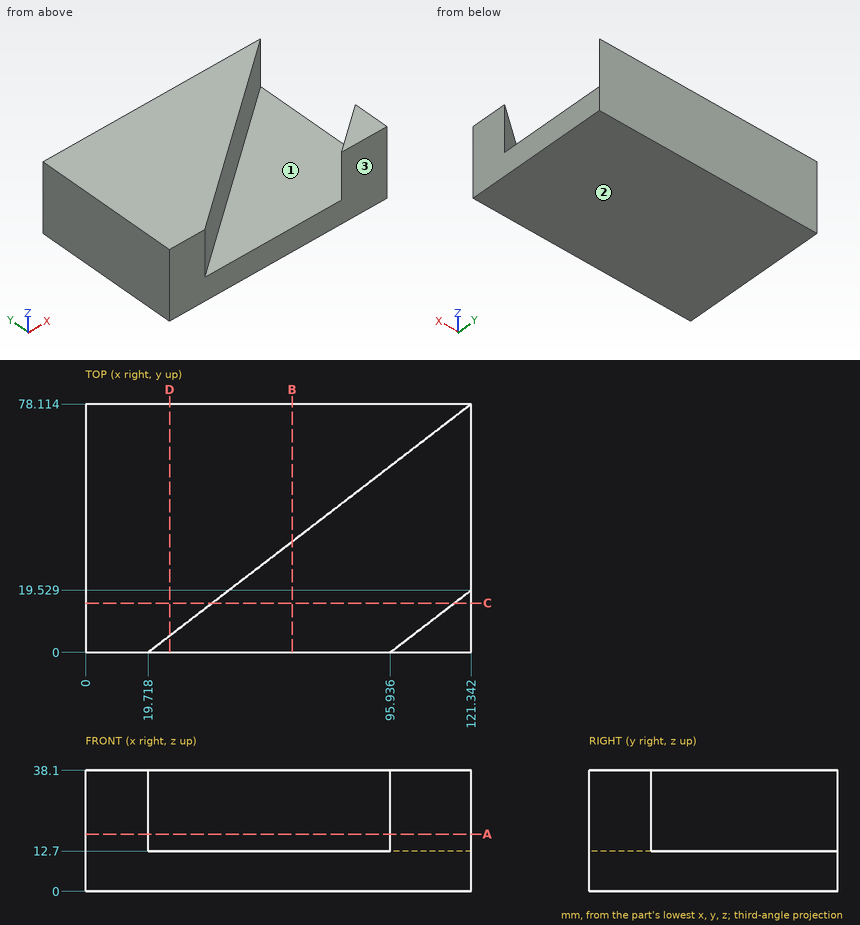
Answer from the drawing. Dimensions are ordinates in mm from the lowest x, y and z of the part. Give positions to 0.01 mm unless a question says otherwise; leave off trailing zeros. Write each loop counter-clockwise with the first axis right and the second up, starting at its lowest first coordinate (ties: lowest second). Pieces come first, ordered by that corner, then holes. Notation, with made-up numbers: (-19.75, 82.25) -> (13.25, 82.25) arc R18 ccw to (13.25, 95.25) -> close; hole circle Ø6 at (12.25, 21.5). An arc over 180 degrees is marked (long way). Use a Markdown table: item, result.
(1) Section C-C, the plane y = 15.5 is taken. Determine the outline of the cut face in (x, z), then the cut area to 3 significant figures.
Return value:
| item | result |
|---|---|
| outline | (0, 0) -> (121.34, 0) -> (121.34, 38.1) -> (116.1, 38.1) -> (116.1, 12.7) -> (39.88, 12.7) -> (39.88, 38.1) -> (0, 38.1) -> close |
| area | 2,690 mm2 |
(2) Section D-D, the plane x = 26.5 is taken. Determine the outline of the cut face in (y, z) (1 decimal).
Return value:
| item | result |
|---|---|
| outline | (0, 0) -> (78.1, 0) -> (78.1, 38.1) -> (5.2, 38.1) -> (5.2, 12.7) -> (0, 12.7) -> close |
(3) A flat-ended cylindrical pin translates along its axis: P1, Ø12, axis at y = 26.5, z = 22.5, coming from the +X side. Find the tip coordinate at first contact, or state that the pin passes through.
Return value:
| item | result |
|---|---|
| P1 | x = 62 |
(4) Determine the mould class of the marked faces 1, 2 and 3 for opening direction Y: released by +Y, released by -Y, zero draft, split by the parting line, or undercut.
Return value:
| item | result |
|---|---|
| face 1 | undercut |
| face 2 | zero draft |
| face 3 | released by -Y |
(5) Find the intervals of material crossed by probe 1 along Z at (x, y) = (111, 36.5); probe 2 along Y at (x, z) = (107, 30.5) (1 decimal); probe 3 along X at (y, z) = (9.5, 29) (1 decimal), in increasing order. Write a range as from..to.
Return value:
| item | result |
|---|---|
| probe 1 | 0..12.7 |
| probe 2 | 0..8.5, 67.1..78.1 |
| probe 3 | 0..32.1, 108.3..121.3 |
(6) Section A-A, the plane z = 18 is taken. Determine the outline of the cut face in (x, y) (1 decimal), then the cut area to 3 significant figures.
Return value:
| item | result |
|---|---|
| outline | (0, 0) -> (19.7, 0) -> (121.3, 78.1) -> (0, 78.1) -> close; (95.9, 0) -> (121.3, 0) -> (121.3, 19.5) -> close |
| area | 5,760 mm2 |
(7) Section B-B, the plane x = 65 is taken. Determine the outline of the cut face in (y, z) (1 decimal), then the cut area to 3 significant figures.
Return value:
| item | result |
|---|---|
| outline | (0, 0) -> (78.1, 0) -> (78.1, 38.1) -> (34.8, 38.1) -> (34.8, 12.7) -> (0, 12.7) -> close |
| area | 2,090 mm2 |
